Check sheet for the modelled part. Datum: model origin and axes. Units: mm. A direction names the side the tool comes from. Round coordinates to 2 decimals unless told otherwise and drop trailing zeros. Order: outer loops, then holes, each group sorted by start corner. A loop starts at its lowest first (then second) coordinate and runs counter-clockwise, first axis right, second up. Notation, with made-up numbers: (28.25, 37.25) -> (78.25, 37.25) arc R27 ccw to (78.25, 65.25) -> close; hole circle Ø7 at (-16, -22). An arc over 180 degrees is marked (long way). Answer in a Markdown table with one row per item. Add a question column.
1. Sectioned sample at B-B, the plane z = -6. Record the boundary of the cut face in (x, y), then the cut area to 4 significant figures.
2. Sectioned sample at A-A, the plane x = 0. Record the boundary of the cut face in (y, z).
3. Sectioned sample at C-C, the plane y = -2. Record the boundary of the cut face in (x, z).
4. Material ranges on L1, parallel to X at y = -0.25, z = 4; L2, parallel to Y at x = -9, z = -4.25; L3, parallel to Y at x = 2.75, z = 0, recorded low to high. Write a range as from..to.
5. Access from +Z, -Z, +X, -X, +Y, -Y to the whole of each face (thin tool, end or side, straight path). Record for faces 1 (the flat face through (0, -2, -0.526)), 2 (the flat face through (0, -2, 7.774)), 3 (the cylindrical face through (-0.443, -5.877, 6.974)), 4 (the flat face through (-4.15, -2, 4)).
6. Sectioned sample at D-D, the plane y = -4.5. Record the boundary of the cut face in (x, z), then the cut area to 3 significant figures.
7. Depth check by flat-ended pin: P1, Ø8, axis at x = 2.5, z = -7.5, coming from the -Y side; P2, Ø5, axis at x = -4, z = -2, coming from the -Y side; P3, Ø0.6, axis at x = 1.5, y = -2, coming from the -Z side. Enter the tip coordinate at first touch or a pass-through.
```python
from build123d import *

# Parameters (mm, degrees)
F0_W     = 25
F0_H     = 23
F1_DEPTH = 1.59
F3_DEPTH = 25
F2_W     = 4.15
F2_H     = 4.15
F2_H_2   = 3.6240464542
F2_H_3   = 0.5259535458
F4_DEPTH = 1.25
F5_R     = 3.4
F6_DEPTH = 6.16
F7_R     = 1


with BuildPart() as f1:
    # F0 (on Front) → F1 (new body)
    with BuildSketch(Plane.XZ):
        Rectangle(F0_W, F0_H)
    extrude(amount=F1_DEPTH)

    # F2 (on face) → F3 (cut)
    with BuildSketch(Plane.XZ.offset(1.59)):
        with BuildLine():
            Line((-10.2684276358, 3.6240464542), (-11.075, 3.6240464542))
            Line((-11.075, 3.6240464542), (-11.075, 2.81747409))
            ThreePointArc((-11.075, 2.81747409), (-10.5046672118, 3.053713666), (-10.2684276358, 3.6240464542))
        make_face()
        with BuildLine():
            ThreePointArc((-10.2684276358, 3.6240464542), (-10.5046672118, 4.1943792424), (-11.075, 4.4306188184))
            Line((-11.075, 4.4306188184), (-11.075, 3.6240464542))
            Line((-11.075, 3.6240464542), (-10.2684276358, 3.6240464542))
        make_face()
        with BuildLine():
            Line((-11.075, 3.6240464542), (-11.075, 4.4306188184))
            ThreePointArc((-11.075, 4.4306188184), (-11.6453327882, 4.1943792424), (-11.8815723642, 3.6240464542))
            Line((-11.8815723642, 3.6240464542), (-11.075, 3.6240464542))
        make_face()
        with BuildLine():
            Line((-11.075, 2.81747409), (-11.075, 3.6240464542))
            Line((-11.075, 3.6240464542), (-11.8815723642, 3.6240464542))
            ThreePointArc((-11.8815723642, 3.6240464542), (-11.6453327882, 3.053713666), (-11.075, 2.81747409))
        make_face()
        with BuildLine():
            Line((-11.075, -10.075), (-11.075, -9.15))
            ThreePointArc((-11.075, -9.15), (-11.7290737726, -9.4209262274), (-12, -10.075))
            Line((-12, -10.075), (-11.075, -10.075))
        make_face()
        with BuildLine():
            Line((-11.075, -10.075), (-10.15, -10.075))
            ThreePointArc((-10.15, -10.075), (-10.4209262274, -9.4209262274), (-11.075, -9.15))
            Line((-11.075, -9.15), (-11.075, -10.075))
        make_face()
        with BuildLine():
            ThreePointArc((-12, -10.075), (-11.075, -11), (-10.15, -10.075))
            Line((-10.15, -10.075), (-11.075, -10.075))
            Line((-11.075, -10.075), (-12, -10.075))
        make_face()
        with BuildLine():
            Line((11.075, -10.075), (10.15, -10.075))
            ThreePointArc((10.15, -10.075), (11.075, -11), (12, -10.075))
            Line((12, -10.075), (11.075, -10.075))
        make_face()
        with BuildLine():
            ThreePointArc((12, -10.075), (11.7290737726, -9.4209262274), (11.075, -9.15))
            Line((11.075, -9.15), (11.075, -10.075))
            Line((11.075, -10.075), (12, -10.075))
        make_face()
        with BuildLine():
            ThreePointArc((11.075, -9.15), (10.4209262274, -9.4209262274), (10.15, -10.075))
            Line((10.15, -10.075), (11.075, -10.075))
            Line((11.075, -10.075), (11.075, -9.15))
        make_face()
        with BuildLine():
            Line((11.075, 2.6990464542), (11.075, 3.6240464542))
            Line((11.075, 3.6240464542), (10.15, 3.6240464542))
            ThreePointArc((10.15, 3.6240464542), (10.4209262274, 2.9699726816), (11.075, 2.6990464542))
        make_face()
        with BuildLine():
            ThreePointArc((12, 3.6240464542), (11.7290737726, 4.2781202268), (11.075, 4.5490464542))
            Line((11.075, 4.5490464542), (11.075, 3.6240464542))
            Line((11.075, 3.6240464542), (12, 3.6240464542))
        make_face()
        with BuildLine():
            Line((12, 3.6240464542), (11.075, 3.6240464542))
            Line((11.075, 3.6240464542), (11.075, 2.6990464542))
            ThreePointArc((11.075, 2.6990464542), (11.7290737726, 2.9699726816), (12, 3.6240464542))
        make_face()
        with BuildLine():
            Line((11.075, 3.6240464542), (11.075, 4.5490464542))
            ThreePointArc((11.075, 4.5490464542), (10.4209262274, 4.2781202268), (10.15, 3.6240464542))
            Line((10.15, 3.6240464542), (11.075, 3.6240464542))
        make_face()
    extrude(amount=-F3_DEPTH, mode=Mode.SUBTRACT)

    # F2 (on face) → F4 (join)
    with BuildSketch(Plane.XZ.offset(1.59)):
        with Locations((-2.075, 5.6990464542)):
            Rectangle(F2_W, F2_H)
        with Locations((2.075, 5.6990464542)):
            Rectangle(F2_W, F2_H)
        with Locations((2.075, 1.8120232271)):
            Rectangle(F2_W, F2_H_2)
        with Locations((-2.075, 1.8120232271)):
            Rectangle(F2_W, F2_H_2)
        with Locations((-2.075, -0.2629767729)):
            Rectangle(F2_W, F2_H_3)
        with Locations((2.075, -0.2629767729)):
            Rectangle(F2_W, F2_H_3)
    extrude(amount=F4_DEPTH)

    # F5 (on face) → F6 (join)
    with BuildSketch(Plane.XZ.offset(2.84)):
        with Locations((0, 3.603294285)):
            Circle(F5_R)
    extrude(amount=F6_DEPTH)

    # F7
    f7_edges = [f1.edges().sort_by_distance(p)[0] for p in [
        (-12.5, -0.795, -11.5),
        (-12.5, -0.795, 11.5),
        (12.5, -0.795, -11.5),
        (12.5, -0.795, 11.5),
    ]]
    fillet(f7_edges, radius=F7_R)


solid = f1.part
```
Answer key:
| question | item | result |
|---|---|---|
| 1 | outline | (-12.5, -1.59) -> (12.5, -1.59) -> (12.5, 0) -> (-12.5, 0) -> close |
| 1 | area | 39.75 mm² |
| 2 | outline | (-9, 0.2) -> (-2.84, 0.2) -> (-2.84, -0.53) -> (-1.59, -0.53) -> (-1.59, -11.5) -> (0, -11.5) -> (0, 11.5) -> (-1.59, 11.5) -> (-1.59, 7.77) -> (-2.84, 7.77) -> (-2.84, 7) -> (-9, 7) -> close |
| 3 | outline | (-4.15, -0.53) -> (4.15, -0.53) -> (4.15, 7.77) -> (-4.15, 7.77) -> close |
| 4 | L1 | x = -12.5..-11.79, -10.36..10.23, 11.92..12.5 |
| 4 | L2 | y = -1.59..0 |
| 4 | L3 | y = -2.84..0 |
| 5 | face 1 | -Z, +X, -X, -Y |
| 5 | face 2 | +Z, +X, -X, -Y |
| 5 | face 3 | -Y |
| 5 | face 4 | +Z, -Z, -X, -Y |
| 6 | outline | circle Ø6.8 at (0, 3.6) |
| 6 | area | 36.3 mm² |
| 7 | P1 | stops at y = -1.59 |
| 7 | P2 | stops at y = -2.84 |
| 7 | P3 | stops at z = -0.53 |
